Check sheet for the modelled part. Datum: model origin and axes. Units: mm. Give positions to 0.01 mm unless a question says otherwise; leave off trailing zeros. Order: outer loops, then holes, each group sorted by start corner. A loop starts at its lowest first (then second) coordinate and runs counter-clockwise, first axis right, second up.
Item 1: Gauge pin test, flat ends, axial feed: P1, Ø3, axis at x = 6.5, y = 151, coming from the +Z side; P2, Ø1.5, axis at y = 70.5, z = 2.5, coming from the +X side; P3, Ø1.4, axis at y = 128.5, z = 2.5, coming from the +X side; P4, Ø3, axis at x = 3.65, y = 137.88, coming from the +Z side. Record the tip position at first contact, or that the pin passes through.
Item 2: Sectioned sample at C-C on x = -45.5. Record the boundary of the cut face in (y, z).
Item 3: Material ranges on line 1 along X through (y, z) = (161, 3.75); line 2 along Y through (x, z) = (-15, 3.75); line 3 along Z through (x, y) = (-2, 126.5), recorded low to high.
Item 4: Sectioned sample at B-B on y = 111.5. Record the boundary of the cut face in (x, z).
Item 5: Sectioned sample at A-A on x = 22. Record the boundary of the cut face in (y, z).
Item 6: Sectioned sample at D-D on y = 91.5. Record the boundary of the cut face in (x, z).
from build123d import *

# Parameters (mm, degrees)
SKETCH2_R               = 84
BOSS_EXTRUDE1_DEPTH     = 3
SKETCH3_R               = 2
CUT_EXTRUDE1_DEPTH      = 3
SKETCH5_W               = 73
SKETCH5_H               = 5
BOSS_EXTRUDE2_DEPTH     = 3
SKETCH6_R               = 2
CUT_EXTRUDE2_DEPTH      = 226.621039578
SKETCH12_W              = 4
SKETCH12_H              = 6
CUT_EXTRUDE3_DEPTH      = 3
FILLET1_R               = 1
BOSS_EXTRUDE3_OUTLINE_R = 3.75
BOSS_EXTRUDE3_DEPTH     = 5
SKETCH16_R              = 2
CUT_EXTRUDE4_DEPTH      = 15.2
CUT_EXTRUDE5_START      = -2
CUT_EXTRUDE5_DEPTH      = 2


# Read off the part's stored shape, not the designer's step: Boss-Extrude3
with BuildPart() as part:
    # Sketch2 → Boss-Extrude1 (new body)
    with BuildSketch(Plane.XY.offset(1)):
        with Locations((3.652326605, 123.87718283)):
            Circle(SKETCH2_R)
    extrude(amount=BOSS_EXTRUDE1_DEPTH)

    # Sketch3 → Cut-Extrude1 (cut)
    with BuildSketch(Plane.XY.offset(4)):
        with BuildLine():
            Line((-2.347673395, 45.105360456), (-2.347673395, 202.649005203))
            ThreePointArc((-2.347673395, 202.649005203), (-75.347673395, 123.87718283), (-2.347673395, 45.105360456))
        make_face()
        with BuildLine():
            Line((9.652326605, 202.649005203), (9.652326605, 45.105360456))
            ThreePointArc((9.652326605, 45.105360456), (61.596265028, 70.178951946), (82.652326605, 123.87718283))
            ThreePointArc((82.652326605, 123.87718283), (61.596265028, 177.575413713), (9.652326605, 202.649005203))
        make_face()
        with Locations((3.652326605, 200.87718283)):
            Circle(SKETCH3_R)
        with Locations((3.652326605, 193.87718283)):
            Circle(SKETCH3_R)
        with Locations((3.652326605, 186.87718283)):
            Circle(SKETCH3_R)
        with Locations((3.652326605, 179.87718283)):
            Circle(SKETCH3_R)
        with Locations((3.652326605, 172.87718283)):
            Circle(SKETCH3_R)
        with Locations((3.652326605, 165.87718283)):
            Circle(SKETCH3_R)
        with Locations((3.652326605, 158.87718283)):
            Circle(SKETCH3_R)
        with Locations((3.652326605, 151.87718283)):
            Circle(SKETCH3_R)
        with Locations((3.652326605, 144.87718283)):
            Circle(SKETCH3_R)
        with Locations((3.652326605, 123.87718283)):
            Circle(SKETCH3_R)
        with Locations((3.652326605, 130.87718283)):
            Circle(SKETCH3_R)
        with Locations((3.652326605, 137.87718283)):
            Circle(SKETCH3_R)
    extrude(amount=-CUT_EXTRUDE1_DEPTH, mode=Mode.SUBTRACT)

    # Sketch5 → Boss-Extrude2 (add)
    with BuildSketch(Plane.XY.offset(4)):
        with Locations((46.152326605, 123.87718283)):
            Rectangle(SKETCH5_W, SKETCH5_H)
        Polygon((4.487263096, 117.431030407), (8.817390114, 119.931030407), (45.317390114, 56.711175931), (40.987263096, 54.211175931), align=None)
        Polygon((-1.512736904, 119.931030407), (2.817390114, 117.431030407), (-33.682609886, 54.211175931), (-38.012736904, 56.711175931), align=None)
        with Locations((-38.847673395, 123.87718283)):
            Rectangle(SKETCH5_W, SKETCH5_H)
        Polygon((2.817390114, 130.323335252), (-1.512736904, 127.823335252), (-38.012736904, 191.043189729), (-33.682609886, 193.543189729), align=None)
        Polygon((8.817390114, 127.823335252), (4.487263096, 130.323335252), (40.987263096, 193.543189729), (45.317390114, 191.043189729), align=None)
    extrude(amount=-BOSS_EXTRUDE2_DEPTH)

    # Sketch6 → Cut-Extrude2 (cut, through all)
    with BuildSketch(Plane.XY.offset(4)):
        with Locations((3.652326605, 130.87718283)):
            Circle(SKETCH6_R)
    extrude(amount=-CUT_EXTRUDE2_DEPTH, mode=Mode.SUBTRACT)

    # Sketch12 → Cut-Extrude3 (cut)
    with BuildSketch(Plane.XY.offset(4)):
        with Locations((3.652326605, 123.87718283)):
            Rectangle(SKETCH12_W, SKETCH12_H)
    extrude(amount=-CUT_EXTRUDE3_DEPTH, mode=Mode.SUBTRACT)

    # Fillet1
    fillet1_edges = [part.edges().sort_by_distance(p)[0] for p in [
        (1.652326605, 120.87718283, 2.5),
        (5.652326605, 126.87718283, 2.5),
        (1.652326605, 126.87718283, 2.5),
        (5.652326605, 120.87718283, 2.5),
    ]]
    fillet(fillet1_edges, radius=FILLET1_R)

    # Boss-Extrude3 outline → Boss-Extrude3 (add)
    with BuildSketch(Plane.XY.offset(4)):
        with BuildLine():
            ThreePointArc((4.48817395, 129.060218544), (3.652326605, 128.87718283), (2.81647926, 129.060218544))
            ThreePointArc((2.81647926, 129.060218544), (3.652326605, 118.62718283), (4.48817395, 129.060218544))
        make_face()
        with Locations((3.652326605, 123.87718283)):
            Circle(BOSS_EXTRUDE3_OUTLINE_R, mode=Mode.SUBTRACT)
    extrude(amount=BOSS_EXTRUDE3_DEPTH)

    # Sketch16 → Cut-Extrude4 (cut)
    with BuildSketch(Plane.XY.offset(16.2)):
        with Locations((3.652326605, 123.87718283)):
            Circle(SKETCH16_R)
    extrude(amount=-CUT_EXTRUDE4_DEPTH, mode=Mode.SUBTRACT)

    # Sketch17 → Cut-Extrude5 (cut)
    with BuildSketch(Plane.XY.offset(16.2).offset(CUT_EXTRUDE5_START)):
        with BuildLine():
            ThreePointArc((2.652326605, 127.491390903), (1.000676176, 126.528833259), (0.038118531, 124.87718283))
            Line((0.038118531, 124.87718283), (1.920275797, 124.87718283))
            ThreePointArc((1.920275797, 124.87718283), (2.238113043, 125.291396392), (2.652326605, 125.609233637))
            Line((2.652326605, 125.609233637), (2.652326605, 127.491390903))
        make_face()
        with BuildLine():
            ThreePointArc((0.038118531, 122.87718283), (1.000676176, 121.2255324), (2.652326605, 120.262974756))
            Line((2.652326605, 120.262974756), (2.652326605, 122.145132022))
            ThreePointArc((2.652326605, 122.145132022), (2.238113043, 122.462969267), (1.920275797, 122.87718283))
            Line((1.920275797, 122.87718283), (0.038118531, 122.87718283))
        make_face()
        with BuildLine():
            Line((4.652326605, 122.145132022), (4.652326605, 120.262974756))
            ThreePointArc((4.652326605, 120.262974756), (6.303977034, 121.2255324), (7.266534679, 122.87718283))
            Line((7.266534679, 122.87718283), (5.384377413, 122.87718283))
            ThreePointArc((5.384377413, 122.87718283), (5.066540167, 122.462969267), (4.652326605, 122.145132022))
        make_face()
        with BuildLine():
            Line((5.384377413, 124.87718283), (7.266534679, 124.87718283))
            ThreePointArc((7.266534679, 124.87718283), (6.303977034, 126.528833259), (4.652326605, 127.491390903))
            Line((4.652326605, 127.491390903), (4.652326605, 125.609233637))
            ThreePointArc((4.652326605, 125.609233637), (5.066540167, 125.291396392), (5.384377413, 124.87718283))
        make_face()
    extrude(amount=CUT_EXTRUDE5_DEPTH, mode=Mode.SUBTRACT)


solid = part.part
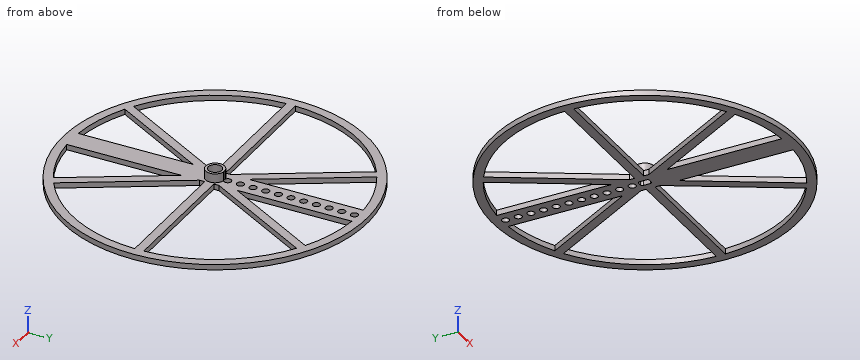
Report:
1. P1: stops at z = 4
1. P2: stops at x = 69.12
1. P3: stops at x = 87.56
1. P4: passes through
2. outline: (55.76, 1) - (62.03, 1) - (62.03, 4) - (55.76, 4) - close; (121.38, 1) - (126.38, 1) - (126.38, 4) - (121.38, 4) - close; (185.72, 1) - (192, 1) - (192, 4) - (185.72, 4) - close
3. line 1: x = -71.7 to -66.08, -20.67 to -14.89, -2.35 to 9.65, 22.2 to 27.97, 73.39 to 79
3. line 2: y = 41.97 to 47.11, 86.57 to 96.57, 121.38 to 126.38, 151.18 to 161.18, 200.64 to 205.78
3. line 3: z = 1 to 4
4. outline: (-79.43, 1) - (-74.37, 1) - (-74.37, 4) - (-79.43, 4) - close; (-6.38, 1) - (13.69, 1) - (13.69, 4) - (-6.38, 4) - close; (81.68, 1) - (86.74, 1) - (86.74, 4) - (81.68, 4) - close
5. outline: (41.91, 1) - (47.04, 1) - (47.04, 4) - (41.91, 4) - close; (87.1, 1) - (97.1, 1) - (97.1, 4) - (87.1, 4) - close; (121.38, 1) - (126.38, 1) - (126.38, 4) - (121.38, 4) - close; (150.66, 1) - (160.66, 1) - (160.66, 4) - (150.66, 4) - close; (200.72, 1) - (205.85, 1) - (205.85, 4) - (200.72, 4) - close
6. outline: (-73.86, 1) - (-68.41, 1) - (-68.41, 4) - (-73.86, 4) - close; (-17.93, 1) - (-12.15, 1) - (-12.15, 4) - (-17.93, 4) - close; (-2.35, 1) - (9.65, 1) - (9.65, 4) - (-2.35, 4) - close; (19.46, 1) - (25.23, 1) - (25.23, 4) - (19.46, 4) - close; (75.71, 1) - (81.16, 1) - (81.16, 4) - (75.71, 4) - close
